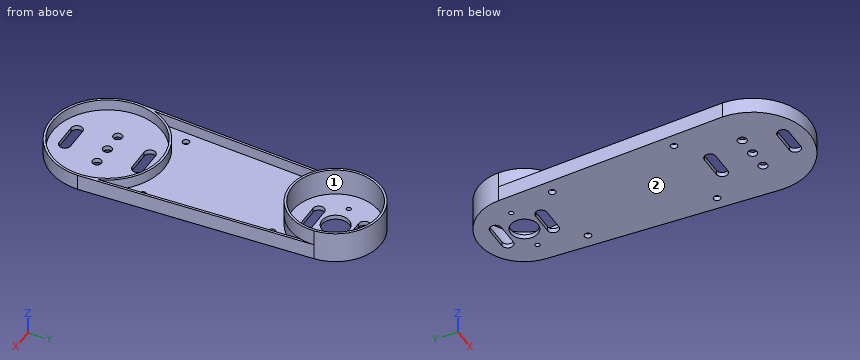
Autodesk Fusion 360 part; units mm, degrees
sketch "스케치1" plane through (0, 0, 0) normal (0, 0, 1) x (1, 0, 0)
  line L0 (19.9753, 100.9938) -> (25, 0)
  line L1 (-19.9753, 100.9938) -> (-25, 0)
  arc A0 (19.9753, 100.9938) -> (-19.9753, 100.9938) centre (0, 100) ccw
  arc A1 (-25, 0) -> (25, 0) centre (0, 0) ccw
  dimension "d1" = 50
  dimension "d222" = 20
  dimension "d223" = 100
extrude "돌출1" add sketch "스케치1" along normal blind 2
sketch "스케치2" plane through (0, 0, 2) normal (0, 0, 1) x (-1, 0, 0)
  arc A0 (-19.9753, -100.9938) -> (19.9753, -100.9938) centre (0, -100) ccw
  line L0 (19.9753, -100.9938) -> (25, 0)
  line L1 (-25, 0) -> (-19.9753, -100.9938)
  line L2 (19.9753, -100.9938) -> (25, 0)
  arc A1 (-19.9753, -100.9938) -> (19.9753, -100.9938) centre (0, -100) ccw
  line L3 (-25, 0) -> (-19.9753, -100.9938)
  arc A2 (25, 0) -> (-25, 0) centre (0, 0) ccw
  line L4 (-23.5864, -8.2873) -> (-19.2868, -94.7068)
  line L5 (19.2868, -94.7068) -> (23.5864, -8.2873)
  circle A3 centre (0, -100) radius 19
  circle A4 centre (0, 0) radius 23.9691
  arc A5 (-23.5864, -8.2873) -> (23.5864, -8.2873) centre (0, 0) ccw
  arc A6 (25, 0) -> (-25, 0) centre (0, 0) ccw
  arc A7 (-19.9753, -100.9938) -> (19.9753, -100.9938) centre (0, -100) ccw
  arc A8 (19.2868, -94.7068) -> (-19.2868, -94.7068) centre (0, -100) ccw
extrude "돌출25" add sketch "스케치2" along normal blind 5
sketch "스케치22" plane through (0, 0, 2) normal (0, 0, 1) x (-1, 0, 0)
  circle A0 centre (0, 0) radius 2
  circle A1 centre (-8.7, 0) radius 2
  circle A2 centre (8.7, 0) radius 2
  circle A3 centre (0, -100) radius 6
  circle A4 centre (-11, -100) radius 1
  circle A5 centre (11, -100) radius 1
  dimension "d208" = 4
  dimension "d209" = 8.7
  dimension "d210" = 8.7
  dimension "d226" = 12
  dimension "d227" = 2
  dimension "d228" = 11
  dimension "d229" = 11
  dimension "d230" = 100
extrude "돌출26" cut sketch "스케치22" against normal blind 2
sketch "스케치24" plane through (0, 0, 7) normal (0, 0, 1) x (-1, 0, 0)
  circle A0 centre (0, -100) radius 20
  circle A1 centre (0, -100) radius 6
  arc A2 (-19.9753, -100.9938) -> (19.9753, -100.9938) centre (0, -100) ccw
  circle A3 centre (0, -100) radius 19
  circle A4 centre (0, -100) radius 19
extrude "돌출28" add sketch "스케치24" along normal blind 7 contours A0 A2
sketch "스케치23" plane through (0, 0, 2) normal (0, 0, 1) x (-1, 0, 0)
  circle A0 centre (-18, -25) radius 1.5
  circle A1 centre (-15, -80) radius 1.5
  circle A2 centre (15, -80) radius 1.5
  circle A3 centre (18, -25) radius 1.5
  circle A4 centre (0, -100) radius 6
  dimension "d214" = 3
  dimension "d215" = 18
  dimension "d216" = 18
  dimension "d217" = 25
  dimension "d225" = 20
  dimension "d233" = 15
  dimension "d234" = 15
extrude "돌출27" cut sketch "스케치23" against normal blind 2 contours A0 | A1 | A2 | A3
sketch "스케치26" plane through (0, 0, 2) normal (0, 0, 1) x (-1, 0, 0)
  line L0 (5, -13.5) -> (-5, -13.5)
  line L1 (5, -18.5) -> (-5, -18.5)
  arc A0 (-5, -13.5) -> (-5, -18.5) centre (-5, -16) ccw
  arc A1 (5, -18.5) -> (5, -13.5) centre (5, -16) ccw
  line L2 (5, 13.5) -> (-5, 13.5)
  line L3 (5, 18.5) -> (-5, 18.5)
  arc A2 (5, 13.5) -> (5, 18.5) centre (5, 16) ccw
  arc A3 (-5, 18.5) -> (-5, 13.5) centre (-5, 16) ccw
  line L4 (5, -112.5) -> (-5, -112.5)
  line L5 (5, -107.5) -> (-5, -107.5)
  arc A4 (5, -112.5) -> (5, -107.5) centre (5, -110) ccw
  arc A5 (-5, -107.5) -> (-5, -112.5) centre (-5, -110) ccw
  line L6 (4.5597, -92.4609) -> (-4.9898, -92.5)
  line L7 (5, -87.5) -> (-5, -87.5)
  arc A6 (4.5597, -92.4609) -> (5, -87.5) centre (5, -90) ccw
  arc A7 (-5, -87.5) -> (-4.9898, -92.5) centre (-5, -90) ccw
  circle A8 centre (0, -100) radius 6
  dimension "d235" = 5
  dimension "d236" = 10
  dimension "d239" = 16
  dimension "d241" = 5
  dimension "d242" = 5
  dimension "d243" = 10
  dimension "d244" = 16
  dimension "d245" = 5
  dimension "d248" = 5
  dimension "d249" = 10
  dimension "d250" = 10
  dimension "d251" = 10
  dimension "d252" = 5
extrude "돌출29" cut sketch "스케치26" against normal blind 2 contours L0 L1 A0 A1 | L2 L3 A2 A3 | L4 L5 A4 A5 | L6 L7 A6 A7
Source: CAD feature listing. Evaluate the final solid. Frame: model axes, mm. Face numbers are marked on the shaded views. Round coordinates to 2 decimals unless told otherwise and drop trailing zeros. Write each loop counter-clockwise with the first axis right and the second up, starting at its lowest first coordinate (ties: lowest second). Pieces come first, ordered by that corner, then holes. Notation, with made-up numbers: M -33.75,32 L -13.75,32 A20 cw -13.75,60 Z; hole C 65,5.5 d1. An arc over 180 degrees is marked long. Use CSV: the item, a comma, the result in double quotes. Start each with the question number.
Q1. Cut plane C-C on z = 10. Output: boundary loops of the cut face in (x, y).
Q2. Cut plane D-D on y = 39. Output: boundary loops of the cut face in (x, z).
Q3. Cut plane B-B on y = -16. Output: boundary loops of the cut face in (x, z).
Q4. Line query: line 1 (Y direction, x = 0, z = 6.75); line 2 (X direction, y = 0, z = 5.65); line 3 (X direction, y = 25, z = 1.3). Output: solid intervals per line, ascending. Write a range as from..to.
Q5. Pull-direction query (Y, two-part tool) for the marked faces 1 and 2; classes: +Y half, -Y half, draft (parallel to the pull), parting line (faces both ways), or undercut.
Q6. First-contact query: P1, Ø3, axis at x = 10.5, y = 34.5, coming from the +Z side; P2, Ø2, axis at y = 25.5, z = 7, coming from the +X side; P3, Ø5, axis at x = -15, z = 5.5, coming from the -Y side. Flat tips, straight axial feed; report the tip coordinate or a pass-through.
Q7. Cut plane A-A on z = 3.25. Output: boundary loops of the cut face in (x, y).
Results found:
1,outline,"C 0,100 d40; hole C 0,100 d38"
2,outline,"M -23.06,0 L 23.06,0 L 23.06,7 L 22.06,7 L 22.06,2 L -22.06,2 L -22.06,7 L -23.06,7 Z"
3,outline,"M -19.21,0 L -7.5,0 L -7.5,2 L -17.85,2 L -17.85,7 L -19.21,7 Z; M 7.5,0 L 19.21,0 L 19.21,7 L 17.85,7 L 17.85,2 L 7.5,2 Z"
4,line 1,"-25..-23.97, 23.97..25, 80..81, 119..120"
4,line 2,"-25..-23.97, 23.97..25"
4,line 3,"-23.76..-19.5, -16.5..16.5, 19.5..23.76"
5,face 1,"undercut"
5,face 2,"draft"
6,P1,"z = 2"
6,P2,"x = 23.78"
6,P3,"y = -21.65"
7,outline,"M -25,0 A25 ccw 25,0 L 19.98,100.99 A20 ccw -19.98,100.99 Z; hole C 0,0 d47.94; hole M -23.59,8.29 A25 cw 23.59,8.29 L 19.29,94.71 A20 cw -19.29,94.71 Z; hole C 0,100 d38"
